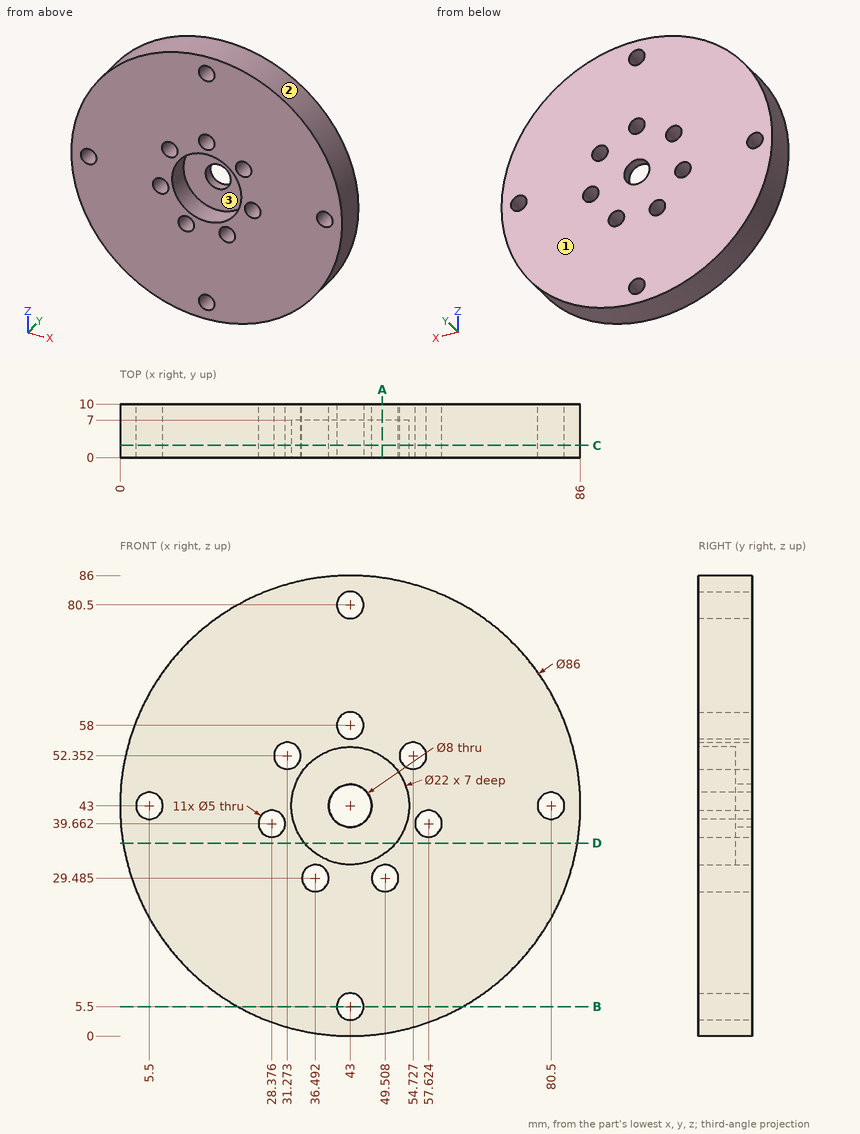
The drawing under review shows one solid part. Ordinate dimensions are in mm from its lowest x, y, z. Coordinates: 2 decimals unless noted, no trailing zeros. Order: outer loops, then holes, each group sorted by start corner. A loop starts at its lowest first (then second) coordinate and runs counter-clockwise, first axis right, second up. Notation, with made-up numbers: (-13, 39) -> (24, 39) arc R11 ccw to (24, 44) -> close; hole circle Ø8 at (72.25, -9.75). An arc over 180 degrees is marked (long way). Use CSV: the item, a comma, the result in double quotes. Start each with the question number.
Item 1: We need section A-A, the plane x = 49. Give the boundary of the cut face in (y, z).
Item 2: Wall thickness on probe 1 along X at (y, z) = (2, 30) (1 decimal); probe 2 along Z at (x, y) = (29.5, 6) (1 decimal); probe 3 along X at (y, z) = (9, 44): over which ranges is each line inside the solid? List them lowest first.
Item 3: We need section D-D, the plane z = 36. Give the boundary of the cut face in (x, y) (1 decimal), then the cut area to 3 significant figures.
Item 4: We need section B-B, the plane z = 5.5. Give the boundary of the cut face in (x, y).
Item 5: Draft analysis for pull direction X (two halves, no side actions). For the marked faces 1, 2 and 3, state which applies: pulls with the +X half, pulls with the -X half, needs draft (parallel to the pull), parting line crosses it, or undercut.
Item 6: Insertion check: pin 1 (8 mm diameter, centred on x = 54.73, z = 52.35, fed in from -Y); pin 2 (6 mm diameter, centred on x = 41, y = 3.5, fed in from -Z); pin 3 (3 mm diameter, centred on x = 66, y = 4.5, fed in from -Z); pin 4 (4.5 mm diameter, centred on x = 43, z = 5.5, fed in from +Y). Each pin has a flat end and moves straight along its axis. Give the tip position at first contact, or say it passes through.
Item 7: We need section C-C, the plane y = 2.25. Give the number of separate pieces and of enclosed holes in the cut face, then the cut area to 3 significant figures.
Derived:
1,outline,"(0, 0.42) -> (10, 0.42) -> (10, 27.04) -> (0, 27.04) -> close; (0, 31.93) -> (10, 31.93) -> (10, 85.58) -> (0, 85.58) -> (0, 52.22) -> (7, 52.22) -> (7, 33.78) -> (0, 33.78) -> close"
2,probe 1,"x = 2 to 34, 38.9 to 47.1, 52 to 84"
2,probe 2,"z = 2.2 to 37.4, 41.9 to 50.6, 54.1 to 83.8"
2,probe 3,"x = 0.01 to 3.21, 7.79 to 39.13, 46.87 to 78.21, 82.79 to 85.99"
3,outline,"(0.6, 0) -> (34.5, 0) -> (34.5, 7) -> (51.5, 7) -> (51.5, 0) -> (85.4, 0) -> (85.4, 10) -> (0.6, 10) -> close"
3,area,"730 mm^2"
4,outline,"(21.96, 0) -> (40.5, 0) -> (40.5, 10) -> (21.96, 10) -> close; (45.5, 0) -> (64.04, 0) -> (64.04, 10) -> (45.5, 10) -> close"
5,face 1,"needs draft"
5,face 2,"parting line crosses it"
5,face 3,"undercut"
6,pin 1,"stops at y = 0"
6,pin 2,"stops at z = 0"
6,pin 3,"stops at z = 5.76"
6,pin 4,"passes through"
7,separate pieces,"1"
7,enclosed holes,"12"
7,area,"5,210 mm^2"
